```python
from build123d import *

# Parameters (mm, degrees)
SKETCH_1_W          = 240
SKETCH_1_H          = 75
EXTRUDE_1_DEPTH     = 1
CHAMFER_1_SIZE      = 10
SKETCH_4_R          = 2.1
SKETCH_4_R_2        = 1.6
CUT_EXTRUDE_3_DEPTH = 10


with BuildPart() as part:
    # 草图1 → 凸台-拉伸1 (new body)
    with BuildSketch(Plane.XY):
        with Locations((120, 37.5)):
            Rectangle(SKETCH_1_W, SKETCH_1_H)
    extrude(amount=EXTRUDE_1_DEPTH)

    # 倒角1
    chamfer_1_edges = [part.edges().sort_by_distance(p)[0] for p in [
        (0, 75, 0.5),
        (240, 75, 0.5),
        (240, 0, 0.5),
        (0, 0, 0.5),
    ]]
    chamfer(chamfer_1_edges, length=CHAMFER_1_SIZE)

    # 草图4 → 切除-拉伸3 (cut)
    with BuildSketch(Plane(origin=(0, 0, 0), x_dir=(-1, 0, 0), z_dir=(0, 0, -1))):
        with Locations((-195, 12)):
            Circle(SKETCH_4_R)
        with Locations((-45, 12)):
            Circle(SKETCH_4_R)
        with Locations((-207.5, 68)):
            Circle(SKETCH_4_R_2)
        with Locations((-192.5, 68)):
            Circle(SKETCH_4_R_2)
        with Locations((-47.5, 68)):
            Circle(SKETCH_4_R_2)
        with Locations((-32.5, 68)):
            Circle(SKETCH_4_R_2)
        with Locations((-235, 37.5)):
            Circle(SKETCH_4_R_2)
        with Locations((-5, 37.5)):
            Circle(SKETCH_4_R_2)
    extrude(amount=-CUT_EXTRUDE_3_DEPTH, mode=Mode.SUBTRACT)


solid = part.part
```
Can you work these out from the model? Positions are in its coordinate system, mm. Give positions to 0.01 mm unless a question says otherwise; leave off trailing zeros. Write item = value, one per line. Start each with the question number.
1. Thinking about a two-plate mould opening in Y: for faces 1 (the face through (118, 38, 1)), 2 (the face through (5.1, 4.9, 0.5)), 3 (the face through (192.997, 12.631, 0.493)), 4 (the face through (234.9, 70.1, 0.5)), which applies, released by +Y, released by -Y, zero draft, split by the parting line, or undercut?
2. For pin 1 (3 mm diameter, centred on x = 207.5, y = 68, fed in from -Z), with a flat end and sliding along its axis, tell me the tip position at first contact or that it passes through.
3. Please list where these lines run through material, in increasing order: line 1 (Y direction, x = 195, z = 0.7); line 2 (Y direction, x = 192.5, z = 0.5); line 3 (X direction, y = 68.5, z = 0.2).
4. Imagine slicing it at A-A (z = 0.25). Count the separate pieces of the cut face and the enclosed holes in it, and give its area (3 significant figures).
Worked answers:
q1.face_1 = zero draft
q1.face_2 = released by -Y
q1.face_3 = undercut
q1.face_4 = released by +Y
q2.pin_1 = through
q3.line_1 = 0 to 9.9, 14.1 to 75
q3.line_2 = 0 to 66.4, 69.6 to 75
q3.line_3 = 3.5 to 30.98, 34.02 to 45.98, 49.02 to 190.98, 194.02 to 205.98, 209.02 to 236.5
q4.separate_pieces = 1
q4.enclosed_holes = 8
q4.area = 17,700 mm2
